Answer from the drawing. Dimensions are ordinates in mm from the lowest x, y and z of the part. Round coordinates to 2 decimals unless told otherwise and drop trailing zeros. Loops run counter-clockwise (first coordinate to the right, second up) from the corner with the lowest first, then second, coordinate; pieces in that order, holes last. Notation, with made-up numbers: (43, 84) - (81, 84) arc R25 ccw to (81, 118) - close; hole circle Ø6 at (45, -17.5). An arc over 180 degrees is marked (long way). Return JSON: item names as keys, results as strings.
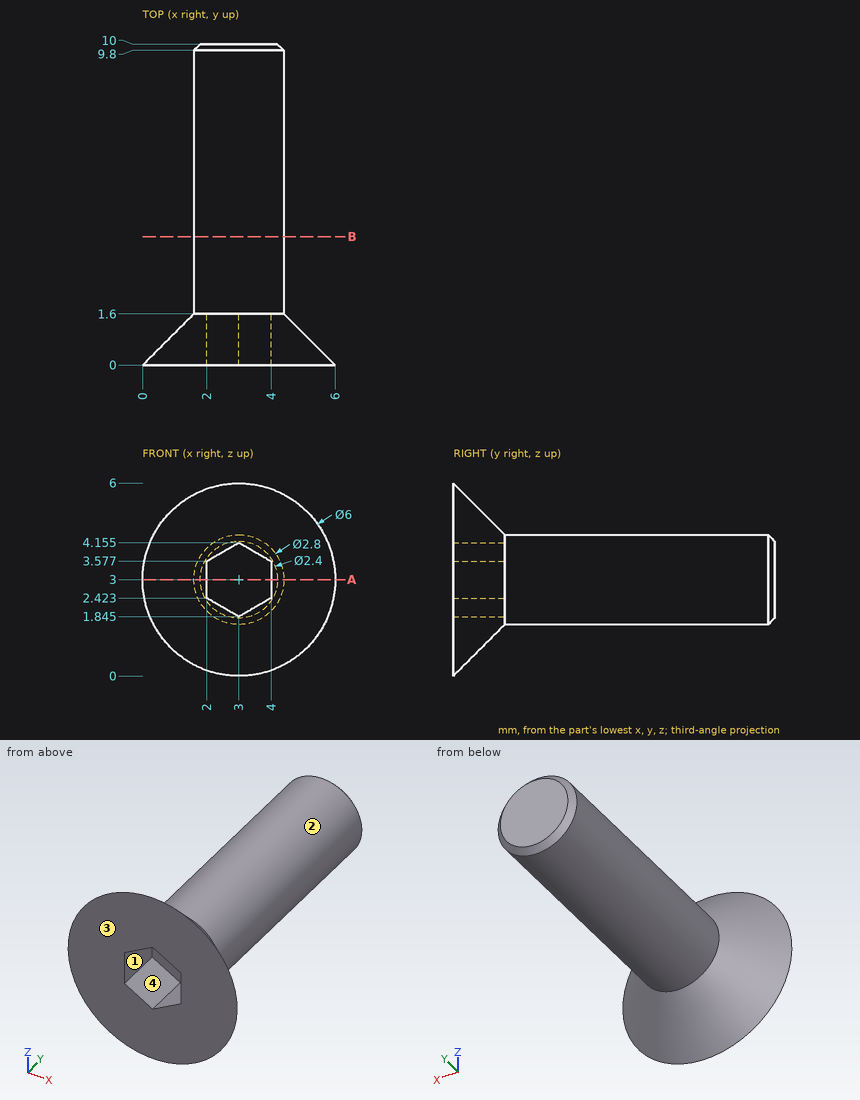
1) Section A-A (z = 3) is taken. Give the vertices of the cut face in (x, y), and give its area (3 significant figures).
Verdict:
{"outline": "(0, 0) - (2, 0) - (2, 1.6) - (4, 1.6) - (4, 0) - (6, 0) - (4.4, 1.6) - (4.4, 9.8) - (4.2, 10) - (1.8, 10) - (1.6, 9.8) - (1.6, 1.6) - close", "area": "27.3 mm2"}
2) Flat-ended cylindrical pins translate along their axes: pin 1 (1 mm diameter, centred on y = 6.5, z = 3, fed in from -X); pin 2 (3 mm diameter, centred on y = 2, z = 4.5, fed in from +X); pin 3 (3 mm diameter, centred on y = 8, z = 1, fed in from +X). Find the tip coordinate at first contact, or state that the pin passes through.
Verdict:
{"pin 1": "stops at x = 1.6", "pin 2": "stops at x = 5.2", "pin 3": "stops at x = 4.31"}
3) Determine the mould class of the marked faces 1, 2, 3 and 4 for opening direction Z: pulls with the +Z half, pulls with the -Z half, needs draft (parallel to the pull), parting line crosses it, or undercut.
Verdict:
{"face 1": "undercut", "face 2": "parting line crosses it", "face 3": "needs draft", "face 4": "undercut"}
4) Find the intervals of material crossed by L1, parallel to Y at x = 2.8, z = 3.4; L2, parallel to Z at x = 2.95, y = 6.75; L3, parallel to X at y = 0.5, z = 2.2 (1 decimal), in increasing order.
Verdict:
{"L1": "y = 1.6 to 10", "L2": "z = 1.6 to 4.4", "L3": "x = 0.6 to 2.4, 3.6 to 5.4"}
5) Section B-B (y = 4) is taken. Give the vertices of the cut face in (x, z).
Verdict:
{"outline": "circle Ø2.8 at (3, 3)"}
